For this review, use the dimensioned drawing (mm, ordinates from the lowest corner) and the shaded views. Round coordinates to 2 decimals unless told otherwise and drop trailing zeros. Write each loop counter-clockwise with the first axis right and the second up, starting at its lowest first coordinate (ties: lowest second). Pieces come first, ordered by that corner, then holes. Notation, with made-up numbers: (-18.75, -36) - (-2.75, -36) arc R22 ccw to (-2.75, -4) - close; hole circle Ø10 at (-30.75, -30). An arc over 180 degrees is marked (long way). Return JSON: item names as keys, results as strings.
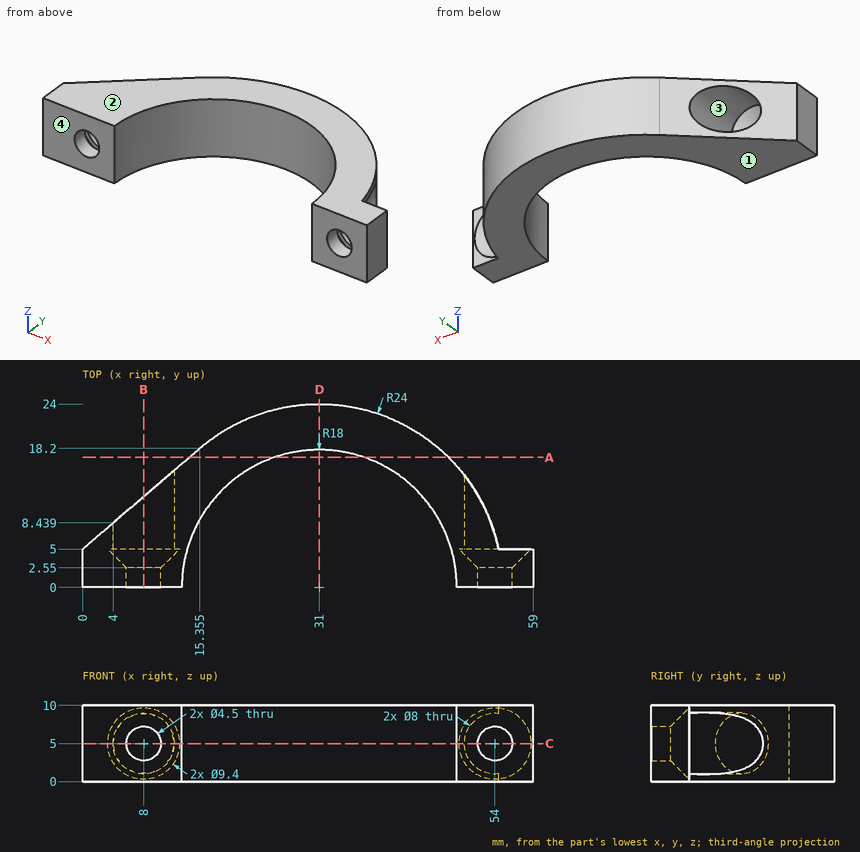
(1) Clearance check with flat-ended pins moving along their axes: pin 1 Ø3 at (x, z) = (32.5, 8.5) entering from -Y; pin 2 Ø1 at (x, z) = (46, 6) entering from +Y (1 decimal); pin 3 Ø5 at (x, z) = (54, 5) entering from +Y. State where each tip first meets the part, or that it passes through.
Filled in:
{"pin 1": "stops at y = 17.75", "pin 2": "stops at y = 19.1", "pin 3": "stops at y = 2.8"}
(2) Add section C-C (z = 5). Give the number of separate pieces and of enclosed holes in the cut face.
Filled in:
{"separate pieces": "3", "enclosed holes": "0"}
(3) Add section D-D (x = 31). Write out the cut boundary in (y, z).
Filled in:
{"outline": "(18, 0) - (24, 0) - (24, 10) - (18, 10) - close"}
(4) Add section B-B (x = 8). Write out the cut boundary in (y, z).
Filled in:
{"outline": "(0, 0) - (11.88, 0) - (11.88, 1) - (5, 1) - (5, 0.3) - (2.55, 2.75) - (0, 2.75) - close; (0, 7.25) - (2.55, 7.25) - (5, 9.7) - (5, 9) - (11.88, 9) - (11.88, 10) - (0, 10) - close"}
(5) Wall thickness on line 1 (Z direction, x = 54, y = 2); line 2 (X direction, y = 7.25, z = 7) (1 decimal); line 3 (X direction, y = 12, z = 4.75) (1 decimal): over which ranges is each line inside the solid? List them lowest first.
Filled in:
{"line 1": "z = 0 to 2.75, 7.25 to 10", "line 2": "x = 2.6 to 4.5, 11.5 to 14.5, 47.5 to 50.5", "line 3": "x = 12 to 17.6, 44.4 to 50"}
(6) Add section A-A (y = 17). Write out the cut boundary in (x, z).
Filled in:
{"outline": "(13.96, 0) - (25.08, 0) - (25.08, 10) - (13.96, 10) - close; (36.92, 0) - (47.94, 0) - (47.94, 10) - (36.92, 10) - close"}
(7) Mouldability with a two-part tool opening along Z and no side actions: class the marked faces 1, 2, 3 and 4 as released by +Z, released by -Z, zero draft, split by the parting line, or undercut.
Filled in:
{"face 1": "released by -Z", "face 2": "released by +Z", "face 3": "undercut", "face 4": "zero draft"}
